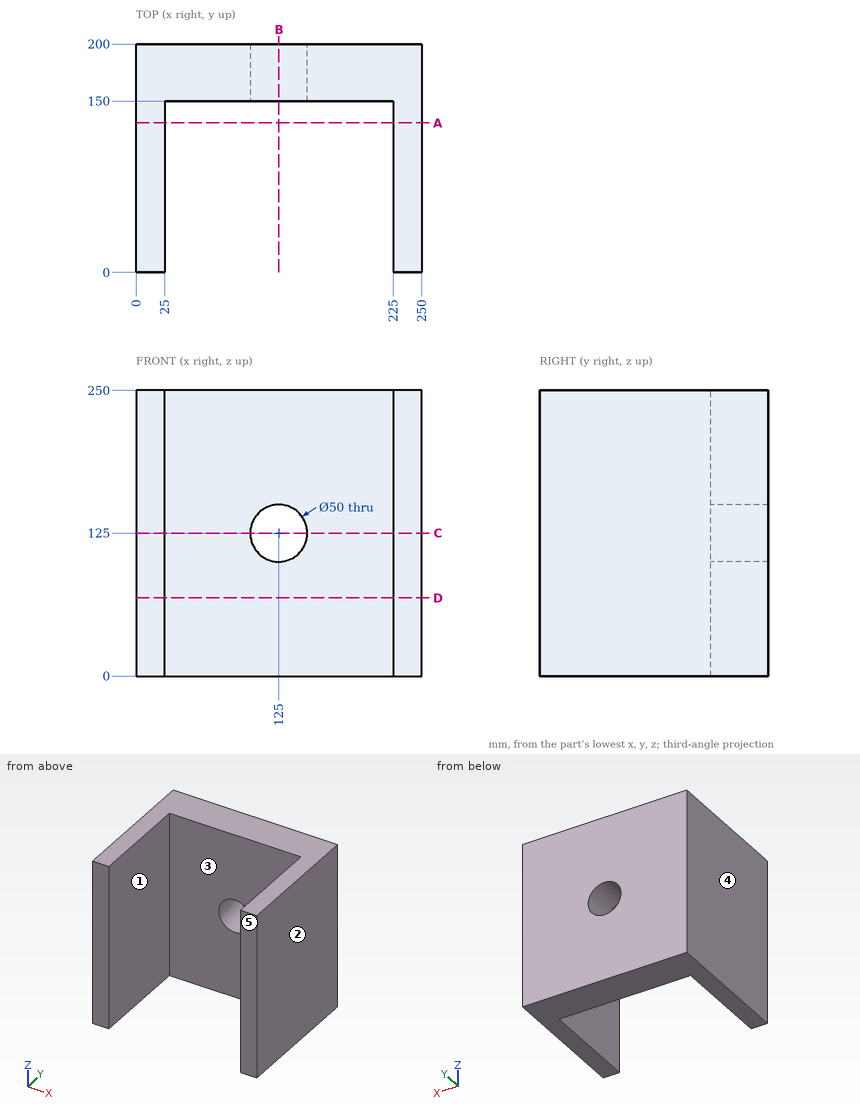
Study the drawing (mm; zero at the part's minimum x, y, z) and answer. A direction names the side the tool comes from. Round coordinates to 2 decimals unless told otherwise and drop trailing zeros. Write each loop counter-clockwise with the first axis right and the second up, starting at its lowest first coordinate (ties: lowest second). Pieces come first, ordered by that corner, then holes.
1) Which of the six approach directions +Z, -Z, +X, -X, +Y, -Y give full straight-line access (tool end or side, diameter ignored) to the marked faces 1 and 2?
2) Consider probe 1 along X at (y, z) = (131, 144.5); probe 2 along Z at (x, y) = (125, 170.5); probe 3 along Y at (x, z) = (159, 55.5). Determine where each line is inside the solid, lowest interval first.
3) Determine the mould class of the marked faces 3, 4 and 5 for opening direction X: pulls with the +X half, pulls with the -X half, needs draft (parallel to the pull), parting line crosses it, or undercut.
4) A flat-ended cylindrical pin translates along its axis: P1, Ø3, axis at x = 195, z = 122.5, coming from the -Y side. Find the tip coordinate at first contact, or state that the pin passes through.
5) A cutting plane is placed at B-B on x = 125. Determine the outline of the cut face in (y, z).
6) A cutting plane is placed at A-A on y = 131. Determine the outline of the cut face in (x, z), and give its area (3 significant figures).
7) A cutting plane is placed at D-D on z = 68.5. Determine the outline of the cut face in (x, y).
8) A cutting plane is placed at C-C on z = 125. Determine the outline of the cut face in (x, y), and give its area (3 significant figures).
Entries:
1. face 1: +Z, -Z, -Y
1. face 2: +Z, -Z, +X, +Y, -Y
2. probe 1: x = 0 to 25, 225 to 250
2. probe 2: z = 0 to 100, 150 to 250
2. probe 3: y = 150 to 200
3. face 3: undercut
3. face 4: pulls with the -X half
3. face 5: needs draft
4. P1: stops at y = 150
5. outline: (150, 0) - (200, 0) - (200, 100) - (150, 100) - close; (150, 150) - (200, 150) - (200, 250) - (150, 250) - close
6. outline: (0, 0) - (25, 0) - (25, 250) - (0, 250) - close; (225, 0) - (250, 0) - (250, 250) - (225, 250) - close
6. area: 12,500 mm2
7. outline: (0, 0) - (25, 0) - (25, 150) - (225, 150) - (225, 0) - (250, 0) - (250, 200) - (0, 200) - close
8. outline: (0, 0) - (25, 0) - (25, 150) - (100, 150) - (100, 200) - (0, 200) - close; (150, 150) - (225, 150) - (225, 0) - (250, 0) - (250, 200) - (150, 200) - close
8. area: 17,500 mm2
